Design review of the part built by this model. Coordinates are the model's own, in mm. A direction names the side the tool comes from. Coordinates: 2 decimals unless noted, no trailing zeros. Order: outer loops, then holes, each group sorted by start corner. A loop starts at its lowest first (then second) coordinate and runs counter-clockwise, first axis right, second up. Notation, with made-up numbers: M 31,18.25 L 56,18.25 A28 ccw 56,57.25 Z; hole C -9.5,2 d7. An arc over 180 degrees is marked long. Use CSV: the item, a comma, the result in double quotes.
```python
from build123d import *

# Parameters (mm, degrees)
F0_R     = 24.847219
F1_DEPTH = 50.8
F2_DEPTH = 12.7
F4_DEPTH = 6.35


with BuildPart() as f1:
    # F0 (on Top) → F1 (new body)
    with BuildSketch(Plane.XY):
        with BuildLine():
            ThreePointArc((99.638521, 0), (80.773834, 31.931442), (43.702941, 30.816859))
            ThreePointArc((43.702941, 30.816859), (26.724861, 0), (43.702941, -30.816859))
            ThreePointArc((43.702941, -30.816859), (80.773834, -31.931442), (99.638521, 0))
        make_face()
        with Locations((63.181691, 0)):
            Circle(F0_R, mode=Mode.SUBTRACT)
    extrude(amount=F1_DEPTH)

    # F0 (on Top) → F2 (join)
    with BuildSketch(Plane.XY):
        with BuildLine():
            Line((43.702941, 30.816859), (-63.181691, 30.816859))
            Line((-63.181691, 30.816859), (-63.181691, -30.816859))
            Line((-63.181691, -30.816859), (43.702941, -30.816859))
            ThreePointArc((43.702941, -30.816859), (26.724861, 0), (43.702941, 30.816859))
        make_face()
    extrude(amount=F2_DEPTH)

    # F3 (on Front) → F4 (join, symmetric)
    with BuildSketch(Plane.XZ):
        Polygon((30.64096, 11.108877), (30.64096, 46.754934), (-22.828124, 11.108877), align=None)
    extrude(amount=F4_DEPTH, both=True)


solid = f1.part
```
(1) Add section D-D on x = 12. State the section outline as (y, z) points, and give its area (3 significant figures).
The answers:
outline,"M -30.82,0 L 30.82,0 L 30.82,12.7 L 6.35,12.7 L 6.35,34.33 L -6.35,34.33 L -6.35,12.7 L -30.82,12.7 Z"
area,"1,060 mm2"
(2) Add section A-A on x = 72.5. State the section outline as (y, z) points, and give its area (3 significant figures).
The answers:
outline,"M -35.25,0 L -23.03,0 L -23.03,50.8 L -35.25,50.8 Z; M 23.03,0 L 35.25,0 L 35.25,50.8 L 23.03,50.8 Z"
area,"1,240 mm2"
(3) Add section B-B on y = 17.5. State the section outline as (x, z) points, and give its area (3 significant figures).
The answers:
outline,"M -63.18,0 L 45.54,0 L 45.54,50.8 L 31.2,50.8 L 31.2,12.7 L -63.18,12.7 Z; M 80.82,0 L 95.16,0 L 95.16,50.8 L 80.82,50.8 Z"
area,"2,660 mm2"
(4) For faces 1 (the face through (14, -6.35, 22)), 2 (the face through (-10, -30.817, 6)), 3 (the face through (-22, 0, 12.7)), 4 (the face through (14, 6.35, 22)), list the 3-axis set-ups (+Z, -Z, +X, -X, +Y, -Y) from which the entire face can be reached by the end or side of a thin tool; tool diameter is ignored.
The answers:
face 1,"+Z, -X, -Y"
face 2,"+Z, -Z, -X, -Y"
face 3,"+Z, -X"
face 4,"+Z, -X, +Y"
(5) Wall thickness on probe 1 along Z at (x, y) = (33.5, -22); probe 2 along X at (y, z) = (12, 43); probe 3 along X at (y, z) = (4, 48.5): over which ranges is each line inside the solid? List them lowest first.
The answers:
probe 1,"z = 0 to 12.7"
probe 2,"x = 28.76 to 41.42, 84.94 to 97.61"
probe 3,"x = 26.94 to 38.66, 87.7 to 99.42"
(6) Clearance check with flat-ended pins moving along their axes: P1, Ø4, axis at x = -22.5, z = 9, coming from the +Y side; P2, Ø4, axis at x = -10, z = 8.5, coming from the -Y side; P3, Ø2, axis at x = 28.5, z = 27, coming from the +Y side. State where each tip first meets the part, or that it passes through.
The answers:
P1,"stops at y = 30.82"
P2,"stops at y = -30.82"
P3,"stops at y = 13.95"
(7) The part is to be moulded in two halves that separate along X. For faces 5 (the face through (-63.182, 0, 6)), 6 (the face through (43.464, -15.119, 25.044)), 7 (the face through (-9, 30.817, 6)), say which applies: pulls with the +X half, pulls with the -X half, needs draft (parallel to the pull), parting line crosses it, or undercut.
The answers:
face 5,"pulls with the -X half"
face 6,"undercut"
face 7,"needs draft"
(8) Add section C-C on z = 23.5. State the section outline as (x, y) points.
The answers:
outline,"M -4.24,-6.35 L 27.28,-6.35 A36.46 ccw 43.7,-30.82 A36.46 ccw long 43.7,30.82 A36.46 ccw 27.28,6.35 L -4.24,6.35 Z; hole C 63.18,0 d49.69"
